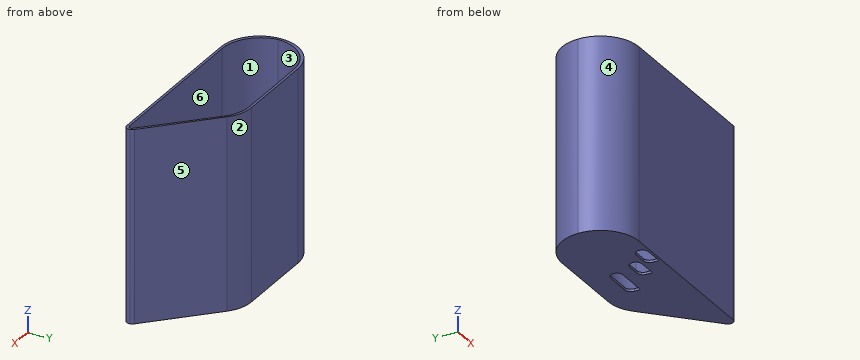
from build123d import *

# Parameters (mm, degrees)
SKETCH1_W               = 85
SKETCH1_H               = 32
BOSS_EXTRUDE1_DEPTH     = 80
CUT_EXTRUDE7_DEPTH      = 122.033053337
CUT_EXTRUDE7_DEPTH_BACK = 80
CUT_EXTRUDE8_DEPTH      = 79
FILLET11_R              = 16
FILLET12_R              = 16
FILLET13_R              = 16
FILLET14_R              = 16
FILLET15_R              = 15
FILLET16_R              = 15
FILLET17_R              = 1.5
FILLET18_R              = 1.5
FILLET21_R              = 3
FILLET22_R              = 2
SKETCH18_W              = 15
SKETCH18_H              = 5
CUT_EXTRUDE14_DEPTH     = 79
SKETCH17_W              = 10
SKETCH17_H              = 5
CUT_EXTRUDE15_DEPTH     = 79
SKETCH16_W              = 10
SKETCH16_H              = 5
CUT_EXTRUDE16_DEPTH     = 79
FILLET29_R              = 2.5
FILLET30_R              = 2.5
FILLET31_R              = 2.5
FILLET32_R              = 2.5
FILLET33_R              = 2.5
FILLET34_R              = 2.5
FILLET35_R              = 2.5
FILLET36_R              = 2.5
FILLET37_R              = 2.5


# Some blends are built 0.0001 mm under size
with BuildPart() as part:
    # Sketch1 → Boss-Extrude1 (new body)
    with BuildSketch(Plane.XY):
        with Locations((42.5, 16)):
            Rectangle(SKETCH1_W, SKETCH1_H)
    extrude(amount=BOSS_EXTRUDE1_DEPTH)

    # Sketch3 → Cut-Extrude7 (cut, two sides: drawn at the far end of the back side and taken through both)
    with BuildSketch(Plane.XY.offset(80).offset(-CUT_EXTRUDE7_DEPTH_BACK)):
        Polygon((221.335887988, -128.791358388), (85, 3), (55, 32), (-81.335887988, 163.791358388), (182.246828788, 436.463134363), (484.918604763, 143.880417587), align=None)
    extrude(amount=CUT_EXTRUDE7_DEPTH + CUT_EXTRUDE7_DEPTH_BACK, mode=Mode.SUBTRACT)

    # Sketch6 → Cut-Extrude8 (cut)
    with BuildSketch(Plane.XY.offset(80)):
        Polygon((1, 31), (1, 1), (84, 1), (84, 2.535105728), (55, 31), align=None)
    extrude(amount=-CUT_EXTRUDE8_DEPTH, mode=Mode.SUBTRACT)

    # Fillet11
    fillet11_edges = [part.edges().sort_by_distance(p)[0] for p in [
        (1, 31, 40.5),
    ]]
    fillet(fillet11_edges, radius=FILLET11_R)

    # Fillet12
    # the kernel refuses this fillet: 16 mm, written as the material it adds along each edge
    with BuildSketch(Plane(origin=(1, 1, 80), x_dir=(0, 1, 0), z_dir=(0, 0, -1))) as fillet12_piece_1:
        with BuildLine():
            CenterArc((16, 15.874507866), FILLET12_R, 180, 82.819244219)
            Line((0, 15.874507866), (-0.32, 15.874507866))
            Line((-0.32, 15.874507866), (-0.32, 0))
            Line((-0.32, 0), (0, -0.32))
            ThreePointArc((0, -0.32), (7, -0.32), (13.96, -0.317490157))
            Line((13.96, -0.317490157), (14, 0))
        make_face()
    extrude(amount=79)

    # Fillet13
    fillet13_edges = [part.edges().sort_by_distance(p)[0] for p in [
        (0, 32, 40),
    ]]
    fillet(fillet13_edges, radius=FILLET13_R)

    # Fillet14
    fillet14_edges = [part.edges().sort_by_distance(p)[0] for p in [
        (0, 0, 40),
    ]]
    fillet(fillet14_edges, radius=FILLET14_R - 0.0001)  # a hair under: the kernel refuses the full size

    # Fillet15
    fillet15_edges = [part.edges().sort_by_distance(p)[0] for p in [
        (55, 31, 40.5),
    ]]
    fillet(fillet15_edges, radius=FILLET15_R)

    # Fillet16
    fillet16_edges = [part.edges().sort_by_distance(p)[0] for p in [
        (55, 32, 40),
    ]]
    fillet(fillet16_edges, radius=FILLET16_R)

    # Fillet17
    fillet17_edges = [part.edges().sort_by_distance(p)[0] for p in [
        (84, 2.535105728, 40.5),
    ]]
    fillet(fillet17_edges, radius=FILLET17_R)

    # Fillet18
    # the kernel refuses this fillet: 1.5 mm, written as the material it adds along each edge
    with BuildSketch(Plane(origin=(84, 1, 80), x_dir=(0, 1, 0), z_dir=(0, 0, -1))) as fillet18_piece_1:
        with BuildLine():
            CenterArc((1.5, -1.377197843), FILLET18_R, 113.345512124, 66.654487876)
            Line((0, -1.377197843), (-0.03, -1.377197843))
            Line((-0.03, -1.377197843), (-0.03, 0))
            Line((-0.03, 0), (0, 0.03))
            ThreePointArc((0, 0.03), (0.4527938, 0.03), (0.893699352, 0.027543957))
            Line((0.893699352, 0.027543957), (0.9055876, 0))
        make_face()
    extrude(amount=79)

    # Fillet21
    fillet21_edges = [part.edges().sort_by_distance(p)[0] for p in [
        (85, 3, 40),
    ]]
    fillet(fillet21_edges, radius=FILLET21_R)

    # Fillet22
    fillet22_edges = [part.edges().sort_by_distance(p)[0] for p in [
        (85, 0, 40),
    ]]
    fillet(fillet22_edges, radius=FILLET22_R)

    # Sketch18 → Cut-Extrude14 (cut)
    with BuildSketch(Plane(origin=(0, 0, 0), x_dir=(-1, 0, 0), z_dir=(0, 0, -1))):
        with Locations((-39.386442529, 20)):
            Rectangle(SKETCH18_W, SKETCH18_H)
    extrude(amount=-CUT_EXTRUDE14_DEPTH, mode=Mode.SUBTRACT)

    # Sketch17 → Cut-Extrude15 (cut)
    with BuildSketch(Plane(origin=(0, 0, 0), x_dir=(-1, 0, 0), z_dir=(0, 0, -1))):
        with Locations((-33.386442529, 10)):
            Rectangle(SKETCH17_W, SKETCH17_H)
    extrude(amount=-CUT_EXTRUDE15_DEPTH, mode=Mode.SUBTRACT)

    # Sketch16 → Cut-Extrude16 (cut)
    with BuildSketch(Plane(origin=(0, 0, 0), x_dir=(-1, 0, 0), z_dir=(0, 0, -1))):
        with Locations((-26.886442529, 3.5)):
            Rectangle(SKETCH16_W, SKETCH16_H)
    extrude(amount=-CUT_EXTRUDE16_DEPTH, mode=Mode.SUBTRACT)

    # Fillet29
    fillet29_edges = [part.edges().sort_by_distance(p)[0] for p in [
        (31.886442529, 22.5, 0.5),
    ]]
    fillet(fillet29_edges, radius=FILLET29_R)

    # Fillet30
    fillet30_edges = [part.edges().sort_by_distance(p)[0] for p in [
        (31.886442529, 17.5, 0.5),
    ]]
    fillet(fillet30_edges, radius=FILLET30_R - 0.0001)  # a hair under: the kernel refuses the full size

    # Fillet31
    fillet31_edges = [part.edges().sort_by_distance(p)[0] for p in [
        (46.886442529, 22.5, 0.5),
    ]]
    fillet(fillet31_edges, radius=FILLET31_R)

    # Fillet32
    fillet32_edges = [part.edges().sort_by_distance(p)[0] for p in [
        (28.386442529, 12.5, 0.5),
    ]]
    fillet(fillet32_edges, radius=FILLET32_R)

    # Fillet33
    fillet33_edges = [part.edges().sort_by_distance(p)[0] for p in [
        (28.386442529, 7.5, 0.5),
    ]]
    fillet(fillet33_edges, radius=FILLET33_R - 0.0001)  # a hair under: the kernel refuses the full size

    # Fillet34
    fillet34_edges = [part.edges().sort_by_distance(p)[0] for p in [
        (38.386442529, 12.5, 0.5),
    ]]
    fillet(fillet34_edges, radius=FILLET34_R)

    # Fillet35
    fillet35_edges = [part.edges().sort_by_distance(p)[0] for p in [
        (21.886442529, 6, 0.5),
    ]]
    fillet(fillet35_edges, radius=FILLET35_R)

    # Fillet36
    fillet36_edges = [part.edges().sort_by_distance(p)[0] for p in [
        (21.886442529, 1, 0.5),
    ]]
    fillet(fillet36_edges, radius=FILLET36_R - 0.0001)  # a hair under: the kernel refuses the full size

    # Fillet37
    fillet37_edges = [part.edges().sort_by_distance(p)[0] for p in [
        (31.886442529, 6, 0.5),
    ]]
    fillet(fillet37_edges, radius=FILLET37_R)


solid = part.part
Verification items for the finished model (mm, model axes). Face numbers are marked on the shaded views. A direction names the side the tool comes from. Coordinates: 2 decimals unless noted, no trailing zeros. Order: outer loops, then holes, each group sorted by start corner. A loop starts at its lowest first (then second) coordinate and runs counter-clockwise, first axis right, second up. Notation, with made-up numbers: M 83.25,-30 L 138.25,-30 A23 ccw 138.25,8 Z; hole C 81,-21.75 d4. An arc over 180 degrees is marked long. One line per item, written item: value. Start each with the question number.
Item 1: Access from +Z, -Z, +X, -X, +Y, -Y to the whole of each face (thin tool, end or side, straight path). Record for the marked faces 5 and 6.
Item 2: Sectioned sample at A-A on x = 50. Record the cut outline in (y, z).
Item 3: Mould release check, pull along Y, two halves, no side actions. Record for the marked faces 1, 2, 3 and 4: pulls with the +Y half, pulls with the -Y half, needs draft (parallel to the pull), parting line crosses it, or undercut.
Item 4: Thickness scan on probe 1 along Y at (x, z) = (21, 10.5); probe 2 along Z at (x, y) = (47, 15); probe 3 along X at (y, z) = (3.5, 40). Record the ranges inside material, lowest first.
Item 5: Depth check by flat-ended pin: P1, Ø8, axis at y = 7.5, z = 44.5, coming from the +X side; P2, Ø2, axis at x = 42.5, y = 11.5, coming from the +Z side; P3, Ø0.5, axis at y = 18, z = 0.5, coming from the -X side; P4, Ø19.5, axis at x = 58.5, z = 46.5, coming from the +Y side. Enter the tip coordinate at first touch or a pass-through.
Item 6: Sectioned sample at B-B on y = 29. Record the cut outline in (x, z), then the cut area to 3 significant figures.
Calculated:
1. face 5: +Z, -Z, +X, +Y
1. face 6: +Z
2. outline: M 0,0 L 31.96,0 L 31.96,80 L 30.96,80 L 30.96,1 L 1,1 L 1,80 L 0,80 Z
3. face 1: undercut
3. face 2: pulls with the +Y half
3. face 3: undercut
3. face 4: pulls with the -Y half
4. probe 1: 0 to 1, 31 to 32
4. probe 2: 0 to 1
4. probe 3: 6.01 to 8.29, 83.02 to 84.42
5. P1: x = 84.42
5. P2: z = 1
5. P3: x = 0.1
5. P4: y = 32
6. outline: M 6.67,0 L 57.94,0 L 57.94,80 L 56.35,80 L 56.35,1 L 9.25,1 L 9.25,80 L 6.67,80 Z
6. area: 380 mm^2
